```python
from build123d import *

# Parameters (mm, degrees)
SKETCH_1_W          = 40
SKETCH_1_H          = 32
EXTRUDE_1_DEPTH     = 12
EXTRUDE_2_DEPTH     = 3
FILLET_1_R          = 10
EXTRUDE_3_DEPTH     = 40
FILLET_2_R          = 10
CUT_EXTRUDE_4_DEPTH = 106.156697477
EXTRUDE_4_DEPTH     = 10
EXTRUDE_5_DEPTH     = 10
EXTRUDE_6_DEPTH     = 10
EXTRUDE_7_DEPTH     = 10
FILLET_3_R          = 3
EXTRUDE_8_DEPTH     = 3
SKETCH_11_W         = 29.594040462
SKETCH_11_H         = 15.509477318
CUT_EXTRUDE_5_DEPTH = 125.135450215


with BuildPart() as part:
    # Эскиз1 → Бобышка-Вытянуть1 (new body)
    with BuildSketch(Plane.XY):
        with Locations((20, 16)):
            Rectangle(SKETCH_1_W, SKETCH_1_H)
    extrude(amount=EXTRUDE_1_DEPTH)

    # Эскиз2 → Бобышка-Вытянуть2 (add)
    with BuildSketch(Plane.XY.offset(12)):
        Polygon((40, 68.92), (9.67, 68.92), (9.67, 61.4), (0, 61.4), (0, 32), (9.67, 32), (40, 32), align=None)
    extrude(amount=-EXTRUDE_2_DEPTH)

    # Скругление1
    # the kernel refuses this fillet: 10 mm, written as the material it adds along each edge
    with BuildSketch(Plane(origin=(0, 32, 9), x_dir=(0, 1, 0), z_dir=(1, 0, 0))) as fillet_1_piece_1:
        with BuildLine():
            CenterArc((9.949874371, -10), FILLET_1_R, 90, 84.260829523)
            Line((0, -9), (-0.198997487, -8.98))
            ThreePointArc((-0.198997487, -8.98), (-0.2, -4.5), (-0.2, 0))
            Line((-0.2, 0), (0, 0.2))
            Line((0, 0.2), (9.949874371, 0.2))
            Line((9.949874371, 0.2), (9.949874371, 0))
        make_face()
    extrude(amount=40)

    # Эскиз3 → Бобышка-Вытянуть3 (add)
    with BuildSketch(Plane.ZY):
        Polygon((-50, 82), (0, 32), (0.953231177, 30.366676535), (6.580561568, 32.490506244), (-44.343145751, 83.414213562), align=None)
    extrude(amount=-EXTRUDE_3_DEPTH)

    # Скругление2
    # the kernel refuses this fillet: 10 mm, written as the material it adds along each edge
    with BuildSketch(Plane(origin=(40, 34.002081727, 5.068986084), x_dir=(0, 0.9816056191455192, 0.19091990064406986), z_dir=(-1, 0, 0))) as fillet_2_piece_1:
        with BuildLine():
            CenterArc((18.680660418, 9.816056191), FILLET_2_R, 146.006473408, 135)
            Line((10.389652956, 15.407048525), (9.56055221, 15.966147758))
            Line((9.56055221, 15.966147758), (-0.829100746, 0.559099233))
            Line((-0.829100746, 0.559099233), (-0.66429077, -0.747474262))
            ThreePointArc((-0.66429077, -0.747474262), (8.743026606, -3.322919186), (20.780779325, -0.981605619))
            Line((20.780779325, -0.981605619), (20.589859424, 0))
        make_face()
    extrude(amount=40)

    # Эскиз5 → Вырез-Вытянуть4 (cut, through all)
    with BuildSketch(Plane(origin=(40, 0, 0), x_dir=(0, 0, -1), z_dir=(1, 0, 0))):
        Polygon((50, 82), (39.176517875, 82), (40.76887279, 85.052981815), (48.441128294, 85.535513608), align=None)
    extrude(amount=-CUT_EXTRUDE_4_DEPTH, mode=Mode.SUBTRACT)

    # Эскиз6 → Бобышка-Вытянуть4 (add)
    with BuildSketch(Plane(origin=(40, 0, 0), x_dir=(0, 0, -1), z_dir=(1, 0, 0))):
        Polygon((34.928932188, 74), (42, 74), (50, 82), (42.928932188, 82), align=None)
    extrude(amount=EXTRUDE_4_DEPTH)

    # Эскиз7 → Бобышка-Вытянуть5 (add)
    with BuildSketch(Plane.ZY):
        Polygon((-42, 74), (-34.928932188, 74), (-42.928932188, 82), (-50, 82), align=None)
    extrude(amount=EXTRUDE_5_DEPTH)

    # Эскиз8 → Бобышка-Вытянуть6 (add)
    with BuildSketch(Plane.ZY.offset(10)):
        Polygon((-42, 74), (-58, 74), (-58, 82), (-50, 82), align=None)
    extrude(amount=-EXTRUDE_6_DEPTH)

    # Эскиз9 → Бобышка-Вытянуть7 (add)
    with BuildSketch(Plane(origin=(50, 0, 0), x_dir=(0, 0, -1), z_dir=(1, 0, 0))):
        Polygon((42, 74), (58, 74), (58, 82), (50, 82), align=None)
    extrude(amount=-EXTRUDE_7_DEPTH)

    # Скругление3
    fillet_3_edges = [part.edges().sort_by_distance(p)[0] for p in [
        (0, 78, -46),
        (40, 78, -46),
    ]]
    fillet(fillet_3_edges, radius=FILLET_3_R)

    # Эскиз10 → Бобышка-Вытянуть8 (add)
    with BuildSketch(Plane(origin=(0, 0, 12), x_dir=(-1, 0, 0), z_dir=(0, 0, -1))):
        with BuildLine():
            Line((-9.67, 91.9), (-2, 91.9))
            Line((-2, 91.9), (-2, 65.4))
            ThreePointArc((-2, 65.4), (-1.472135955, 63.163932023), (0, 61.4))
            Line((0, 61.4), (-9.67, 61.4))
            Line((-9.67, 61.4), (-9.67, 91.9))
        make_face()
    extrude(amount=EXTRUDE_8_DEPTH)

    # Эскиз11 → Вырез-Вытянуть5 (cut, through all)
    with BuildSketch(Plane(origin=(50, 0, 0), x_dir=(0, 0, -1), z_dir=(1, 0, 0))):
        with Locations((46.795384827, 80.754738659)):
            Rectangle(SKETCH_11_W, SKETCH_11_H)
    extrude(amount=-CUT_EXTRUDE_5_DEPTH, mode=Mode.SUBTRACT)


solid = part.part
```
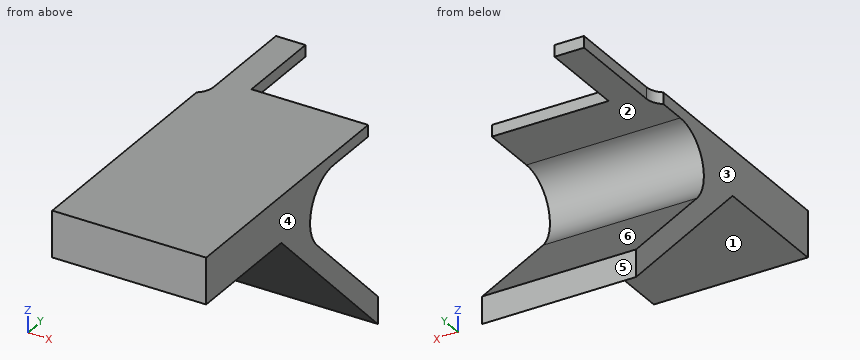
Build history of the part. All positions in model axes, mm. Face numbers are marked on the shaded views. A direction names the side the tool comes from. Round coordinates to 2 decimals unless told otherwise and drop trailing zeros. Write each loop counter-clockwise with the first axis right and the second up, starting at its lowest first coordinate (ties: lowest second). Pieces come first, ordered by that corner, then holes. Notation, with made-up numbers: (65.5, -18) - (119.5, -18) arc R15 cw to (119.5, -8) - close; hole circle Ø10 at (-21, 4). An arc over 180 degrees is marked (long way). Answer as CSV lines item,"result".
Q1. Drop flat-ended pins along their axis: pin 1 (2 mm diameter, centred on x = 19.5, z = 0, fed in from +Y); pin 2 (2.5 mm diameter, centred on y = 83.5, z = 10, fed in from -X); pin 3 (6 mm diameter, centred on x = 11.5, y = 64, fed in from -Z); pin 4 (2 mm diameter, centred on x = 34, z = 3, fed in from -Y). Give the stop position or say it passes through.
Report:
pin 1,"stops at y = 44.42"
pin 2,"stops at x = 2"
pin 3,"stops at z = -35"
pin 4,"stops at y = 0"
Q2. Cut at B-B (x = 4). Write the cut outline in (y, z), and give its area (3 significant figures).
Report:
outline,"(0, 0) - (32, 0) - (73, -41) - (73, -33.93) - (47.14, -8.07) arc R10 cw to (54.21, 9) - (91.9, 9) - (91.9, 12) - (0, 12) - close"
area,"975 mm^2"
Q3. Drill centre lines: probe 1 along Z at (x, y) = (20.5, 65); probe 2 along Z at (x, y) = (18, 20); probe 3 along Z at (x, y) = (12, 51). Where is each one in solid material? Low to high. Write a range as [from, to].
Report:
probe 1,"z = [-33, -25.93], [9, 12]"
probe 2,"z = [0, 12]"
probe 3,"z = [-19, -11.93], [8.47, 12]"
Q4. Cut at D-D (x = 27.5). Write the cut outline in (y, z), and give its area (3 significant figures).
Report:
outline,"(0, 0) - (32, 0) - (73, -41) - (73, -33.93) - (47.14, -8.07) arc R10 cw to (54.21, 9) - (68.92, 9) - (68.92, 12) - (0, 12) - close"
area,"906 mm^2"
Q5. Pull direction Z, two halves, no side cores. Call the marked faces 1, 2 and 3: +Z half, -Z half, draft (parallel to the pull), parting line (faces both ways), or undercut.
Report:
face 1,"-Z half"
face 2,"undercut"
face 3,"draft"
Q6. Cut at A-A (y = 53). Write the cut outline in (x, z).
Report:
outline,"(0, -21) - (40, -21) - (40, -13.93) - (0, -13.93) - close; (0, 8.93) - (40, 8.93) - (40, 12) - (0, 12) - close"
Q7. Tool access for the marked faces 4, 5 and 6: list every direction of +Z, -Z, +X, -X, +Y, -Y with a clear straight run to the whole face (end or side of a thin tool).
Report:
face 4,"+Z, -Z, +X, +Y, -Y"
face 5,"-Z, +X, -X, +Y"
face 6,"+X, -X, +Y"
Q8. Cut at C-C (y = 72). Write the cut outline in (x, z), and give its area (3 significant figures).
Report:
outline,"(0, -40) - (40, -40) - (40, -32.93) - (0, -32.93) - close; (2, 9) - (9.67, 9) - (9.67, 12) - (2, 12) - close"
area,"306 mm^2"
